from build123d import *

# Parameters (mm, degrees)
F0_R     = 4.25
F1_DEPTH = 3
F2_R     = 5.75
F3_DEPTH = 1
F4_R     = 11
F5_DEPTH = 2
F6_R     = 0.5


with BuildPart() as f1:
    # F0 (on Top) → F1 (new body)
    with BuildSketch(Plane.XY):
        Circle(F0_R)
    extrude(amount=F1_DEPTH)

    # F2 (on face) → F3 (join)
    with BuildSketch(Plane.XY.offset(3)):
        Circle(F2_R)
    extrude(amount=F3_DEPTH)

    # F4 (on face) → F5 (join)
    with BuildSketch(Plane.XY.offset(4)):
        Circle(F4_R)
    extrude(amount=F5_DEPTH)

    # F6
    f6_edges = [f1.edges().sort_by_distance(p)[0] for p in [
        (-11, 0, 6),
    ]]
    fillet(f6_edges, radius=F6_R)


solid = f1.part
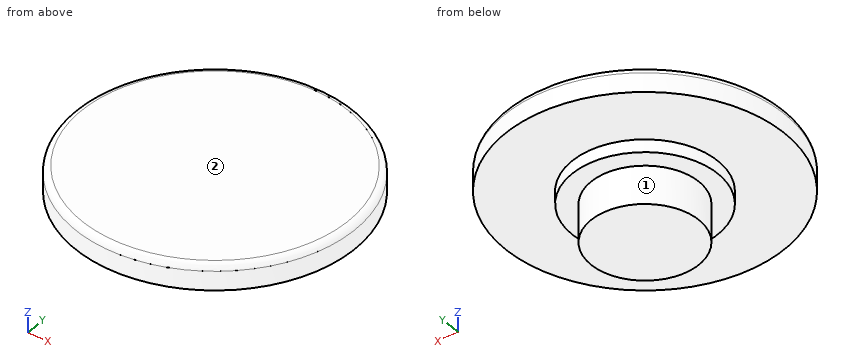
Read the model definition and answer for the solid it produces. Units are mm, in the model's axes. Face numbers are marked on the shaded views. A direction names the side the tool comes from. Coordinates: 2 decimals unless noted, no trailing zeros. Loops run counter-clockwise (first coordinate to the right, second up) from the corner with the lowest first, then second, coordinate; pieces in that order, holes last.
Q1. The part is cut by section D-D on z = 1.2. Write down the section's boundary in (x, y).
Q2. The part is cut by section A-A on y = 0. Write down the section's boundary in (x, z), and give its area (3 significant figures).
Q3. Which of the six approach directions +Z, -Z, +X, -X, +Y, -Y give full straight-line access (tool end or side, diameter ignored) to the marked faces 1 and 2?
Q4. Each of these flat-tipped pins is pushed along its axis until it touches: pin 1 Ø3 at (x, z) = (5.5, 4) entering from -Y; pin 2 Ø2 at (x, z) = (6.5, 4) entering from +Y; pin 3 Ø1.5 at (x, z) = (-8.5, 5) entering from -Y. Where does it stop, or does it pass through?
Q5. Consider probe 1 along Z at (x, y) = (-7.5, 3.5); probe 2 along Z at (x, y) = (-2.75, -4.75); probe 3 along Y at (x, z) = (0.5, 1.45). Determine where each line is inside the solid, lowest interval first.
Q6. The part is cut by section C-C on z = 3.6. Write down the section's boundary in (x, y).
Results below:
1. outline: circle Ø8.5 at (0, 0)
2. outline: (-11, 4) - (-5.75, 4) - (-5.75, 3) - (-4.25, 3) - (-4.25, 0) - (4.25, 0) - (4.25, 3) - (5.75, 3) - (5.75, 4) - (11, 4) - (11, 5.5) arc R0.5 ccw to (10.5, 6) - (-10.5, 6) arc R0.5 ccw to (-11, 5.5) - close
2. area: 80.9 mm2
3. face 1: -Z
3. face 2: +Z, +X, -X, +Y, -Y
4. pin 1: stops at y = -10.25
4. pin 2: stops at y = 9.53
4. pin 3: stops at y = -7.81
5. probe 1: z = 4 to 6
5. probe 2: z = 3 to 6
5. probe 3: y = -4.22 to 4.22
6. outline: circle Ø11.5 at (0, 0)
